Source: CAD feature listing. Evaluate the final solid. Frame: model axes, mm. Face numbers are marked on the shaded views. A direction names the side the tool comes from. Round coordinates to 2 decimals unless told otherwise and drop trailing zeros. Write each loop counter-clockwise with the first axis right and the second up, starting at its lowest first coordinate (ties: lowest second). Pieces come first, ordered by that corner, then holes. Notation, with made-up numbers: M 38.5,54 L 55.5,54 A19 cw 55.5,71 Z; hole C 2.5,13 d2. An arc over 180 degrees is marked long. Answer in a Markdown table with one row per item.
from build123d import *

# Parameters (mm, degrees)
SENSOR_BODY_BASE_DEPTH            = 9
CAMERA_HOLE_SKETCH_R              = 5.25
CAMERA_HOLE_DEPTH                 = 55.697637212
COVER_PLATE_CUTOUT_DEPTH          = 2
LED_DRIVER_CUTOUT_DEPTH           = 55.40433362
LED_DRIVER_CUTOUT_DEPTH_BACK      = 4
LEAD_START                        = 55.40433362
LEAD_CUTOUT_DEPTH                 = 62.40433362
FOLDED_LEAD_CUTOUT_DEPTH          = 4
GREEN_LEAD_CUTOUT_SKETCH_W        = 4
GREEN_LEAD_CUTOUT_SKETCH_H        = 6
GREEN_LEAD_CUTOUT_DEPTH           = 55.40433362
FOLDED_GREEN_LEAD_CUTOUT_SKETCH_W = 4.025
FOLDED_GREEN_LEAD_CUTOUT_SKETCH_H = 6
FOLDED_GREEN_LEAD_CUTOUT_DEPTH    = 4
CAMERA_PCB_CUTOUT_DEPTH           = 1.69
COVER_START                       = 1.69
COVER_PLATE_SUPPORT_DEPTH         = 1.69


with BuildPart() as part:
    # Sensor Body Base Sketch → Sensor Body Base (new body)
    with BuildSketch(Plane(origin=(0, 0, 0), x_dir=(1, 0, 0), z_dir=(0, 1, 0))):
        with BuildLine():
            Line((0, 17.5294293), (51.025, 17.5294293))
            Line((51.025, 17.5294293), (51.025, -17.5294293))
            Line((51.025, -17.5294293), (0, -17.5294293))
            ThreePointArc((0, -17.5294293), (-17.5294293, 0), (0, 17.5294293))
        make_face()
    extrude(amount=SENSOR_BODY_BASE_DEPTH)

    # Camera Hole Sketch → Camera Hole (cut, through all)
    with BuildSketch(Plane(origin=(0, 9, 0), x_dir=(1, 0, 0), z_dir=(0, 1, 0))):
        with Locations(Location((0, 0, 0), (0, 0, 270))):
            Circle(CAMERA_HOLE_SKETCH_R)
    extrude(amount=-CAMERA_HOLE_DEPTH, mode=Mode.SUBTRACT)

    # Cover Plate Cutout Sketch → Cover Plate Cutout (cut)
    # profile 1 of 2: a face of its own
    with BuildSketch(Plane(origin=(0, 9, 0), x_dir=(1, 0, 0), z_dir=(0, 1, 0))):
        with BuildLine():
            Line((47.325, 15.29), (0, 15.29))
            ThreePointArc((0, 15.29), (-15.29, 0), (0, -15.29))
            Line((0, -15.29), (47.325, -15.29))
            Line((47.325, -15.29), (47.325, -5.29))
            Line((47.325, -5.29), (47.325, 5.29))
            Line((47.325, 5.29), (47.325, 15.29))
        make_face()
        with BuildLine():
            ThreePointArc((4.308421985, -3), (-5.25, 0), (4.308421985, 3))
            Line((4.308421985, 3), (10.72655949, 3))
            Line((10.72655949, 3), (10.72655949, -3))
            Line((10.72655949, -3), (4.308421985, -3))
        make_face(mode=Mode.SUBTRACT)
    # profile 2 of 2: a face of its own
    with BuildSketch(Plane(origin=(0, 9, 0), x_dir=(1, 0, 0), z_dir=(0, 1, 0))):
        with BuildLine():
            Line((10.72655949, 3), (4.308421985, 3))
            ThreePointArc((4.308421985, 3), (5.009077531, 1.57214576), (5.25, 0))
            ThreePointArc((5.25, 0), (5.009077531, -1.57214576), (4.308421985, -3))
            Line((4.308421985, -3), (10.72655949, -3))
            Line((10.72655949, -3), (10.72655949, 3))
        make_face()
    extrude(amount=-COVER_PLATE_CUTOUT_DEPTH, mode=Mode.SUBTRACT)

    # LED Driver Cutout Sketch → LED Driver Cutout (cut, two sides: drawn at the far end of the back side and taken through both)
    with BuildSketch(Plane(origin=(0, 7, 0), x_dir=(1, 0, 0), z_dir=(0, 1, 0)).offset(-LED_DRIVER_CUTOUT_DEPTH_BACK)):
        Polygon((36.725, -17.5294293), (47.325, -17.5294293), (47.325, 17.5294293), (38.225, 17.5294293), (38.225, 15.29), (20.025, 15.29), (20.025, -15.29), (36.725, -15.29), align=None)
    extrude(amount=LED_DRIVER_CUTOUT_DEPTH + LED_DRIVER_CUTOUT_DEPTH_BACK, mode=Mode.SUBTRACT)

    # Cover Plate Fastener Sketch → Cover Plate Fastener (revolve, cut)
    with BuildSketch(Plane.XY, mode=Mode.PRIVATE) as cover_plate_fastener_sk:
        Polygon((8.5, 7), (8.5, 3.213974596), (10, 4.08), (10, 7), align=None)
    revolve(cover_plate_fastener_sk.sketch.rotate(Axis((8.5, 7, 0), (0, -1, 0)), 90), axis=Axis((8.5, 7, 0), (0, -1, 0)), mode=Mode.SUBTRACT)

    # Lead Cutout Shared Sketch → Lead Cutout (cut)
    with BuildSketch(Plane(origin=(0, 7, 0), x_dir=(1, 0, 0), z_dir=(0, 1, 0)).offset(LEAD_START)):
        with BuildLine():
            ThreePointArc((0, -13.5294293), (-6.76471465, -11.716829473), (-11.716829473, -6.76471465))
            Line((-11.716829473, -6.76471465), (-13.241528424, -7.645))
            ThreePointArc((-13.241528424, -7.645), (-7.645, -13.241528424), (0, -15.29))
            Line((0, -15.29), (11.279002615, -15.29))
            ThreePointArc((11.279002615, -15.29), (12.340917186, -14.446513871), (13.339960375, -13.5294293))
            Line((13.339960375, -13.5294293), (10.025, -13.5294293))
            Line((10.025, -13.5294293), (0, -13.5294293))
        make_face()
    lead_cutout = extrude(amount=-LEAD_CUTOUT_DEPTH, mode=Mode.SUBTRACT)

    # Sketch11<5> → Folded Lead Cutout (cut)
    with BuildSketch(Plane(origin=(0, 7, 0), x_dir=(1, 0, 0), z_dir=(0, 1, 0))):
        with BuildLine():
            Line((10.025, -4), (10.025, -13.5294293))
            Line((10.025, -13.5294293), (13.339960375, -13.5294293))
            ThreePointArc((13.339960375, -13.5294293), (13.687104196, -13.178132597), (14.025, -12.817931775))
            Line((14.025, -12.817931775), (14.025, -8))
            Line((14.025, -8), (20.025, -8))
            Line((20.025, -8), (20.025, -4))
            Line((20.025, -4), (10.025, -4))
        make_face()
    folded_lead_cutout = extrude(amount=-FOLDED_LEAD_CUTOUT_DEPTH, mode=Mode.SUBTRACT)

    # Lead Cutout Mirror: Lead Cutout, Folded Lead Cutout across plane
    add(lead_cutout.mirror(Plane.XY), mode=Mode.SUBTRACT)
    add(folded_lead_cutout.mirror(Plane.XY), mode=Mode.SUBTRACT)

    # Green Lead Cutout Sketch → Green Lead Cutout (cut, through all)
    with BuildSketch(Plane(origin=(0, 7, 0), x_dir=(1, 0, 0), z_dir=(0, 1, 0))):
        with Locations((14, 0)):
            Rectangle(GREEN_LEAD_CUTOUT_SKETCH_W, GREEN_LEAD_CUTOUT_SKETCH_H)
    extrude(amount=-GREEN_LEAD_CUTOUT_DEPTH, mode=Mode.SUBTRACT)

    # Folded Green Lead Cutout Sketch → Folded Green Lead Cutout (cut)
    with BuildSketch(Plane(origin=(0, 7, 0), x_dir=(1, 0, 0), z_dir=(0, 1, 0))):
        with Locations((18.0125, 0)):
            Rectangle(FOLDED_GREEN_LEAD_CUTOUT_SKETCH_W, FOLDED_GREEN_LEAD_CUTOUT_SKETCH_H)
    extrude(amount=-FOLDED_GREEN_LEAD_CUTOUT_DEPTH, mode=Mode.SUBTRACT)

    # Camera PCB Cutout Sketch → Camera PCB Cutout (cut)
    with BuildSketch(Plane(origin=(0, 7, 0), x_dir=(1, 0, 0), z_dir=(0, 1, 0))):
        with BuildLine():
            Line((-11.716829473, 6.76471465), (-13.241528424, 7.645))
            ThreePointArc((-13.241528424, 7.645), (-15.29, 0), (-13.241528424, -7.645))
            Line((-13.241528424, -7.645), (-11.716829473, -6.76471465))
            ThreePointArc((-11.716829473, -6.76471465), (-6.76471465, -11.716829473), (0, -13.5294293))
            Line((0, -13.5294293), (10.025, -13.5294293))
            Line((10.025, -13.5294293), (10.025, -4.5))
            Line((10.025, -4.5), (4.5, -4.5))
            Line((4.5, -4.5), (2.704163457, -4.5))
            ThreePointArc((2.704163457, -4.5), (0, -5.25), (-2.704163457, -4.5))
            Line((-2.704163457, -4.5), (-4.5, -4.5))
            Line((-4.5, -4.5), (-4.5, -2.704163457))
            ThreePointArc((-4.5, -2.704163457), (-5.25, 0), (-4.5, 2.704163457))
            Line((-4.5, 2.704163457), (-4.5, 4.5))
            Line((-4.5, 4.5), (-2.704163457, 4.5))
            ThreePointArc((-2.704163457, 4.5), (0, 5.25), (2.704163457, 4.5))
            Line((2.704163457, 4.5), (4.5, 4.5))
            Line((4.5, 4.5), (10.025, 4.5))
            Line((10.025, 4.5), (10.025, 13.5294293))
            Line((10.025, 13.5294293), (0, 13.5294293))
            ThreePointArc((0, 13.5294293), (-6.76471465, 11.716829473), (-11.716829473, 6.76471465))
        make_face()
        with BuildLine():
            Line((4.5, -4.5), (4.5, -2.704163457))
            ThreePointArc((4.5, -2.704163457), (3.712310601, -3.712310601), (2.704163457, -4.5))
            Line((2.704163457, -4.5), (4.5, -4.5))
        make_face()
        with BuildLine():
            ThreePointArc((-2.704163457, -4.5), (-3.712310601, -3.712310601), (-4.5, -2.704163457))
            Line((-4.5, -2.704163457), (-4.5, -4.5))
            Line((-4.5, -4.5), (-2.704163457, -4.5))
        make_face()
        with BuildLine():
            ThreePointArc((-4.5, 2.704163457), (-3.712310601, 3.712310601), (-2.704163457, 4.5))
            Line((-2.704163457, 4.5), (-4.5, 4.5))
            Line((-4.5, 4.5), (-4.5, 2.704163457))
        make_face()
        with BuildLine():
            Line((4.5, 2.704163457), (4.5, 4.5))
            Line((4.5, 4.5), (2.704163457, 4.5))
            ThreePointArc((2.704163457, 4.5), (3.712310601, 3.712310601), (4.5, 2.704163457))
        make_face()
    extrude(amount=-CAMERA_PCB_CUTOUT_DEPTH, mode=Mode.SUBTRACT)

    # Cover Plate Support Sketch → Cover Plate Support (add)
    with BuildSketch(Plane(origin=(0, 5.31, 0), x_dir=(1, 0, 0), z_dir=(0, 1, 0)).offset(COVER_START)):
        with BuildLine():
            Line((-11.716829473, 6.76471465), (-13.241528424, 7.645))
            ThreePointArc((-13.241528424, 7.645), (-15.29, 0), (-13.241528424, -7.645))
            Line((-13.241528424, -7.645), (-11.716829473, -6.76471465))
            ThreePointArc((-11.716829473, -6.76471465), (-13.5294293, 0), (-11.716829473, 6.76471465))
        make_face()
    extrude(amount=-COVER_PLATE_SUPPORT_DEPTH)


solid = part.part
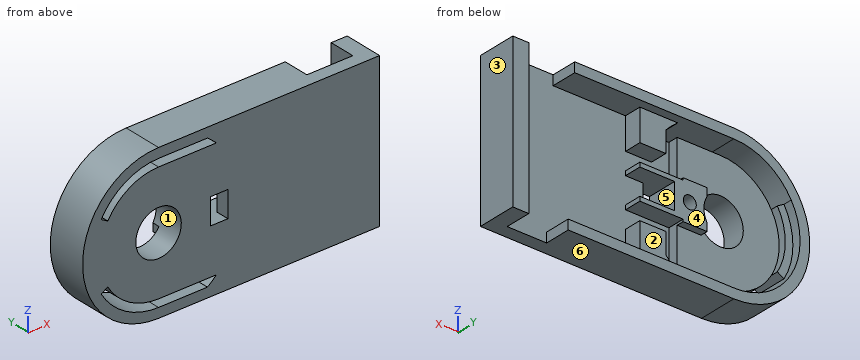
Q1. Access query for the marked faces 1 and 2. Directions: +Z, -Z, +X, -X, +Y, -Y. A direction counts if a zero-diameter tool reaches every point of the face in a straight line with its end or side. Return the directions, or none.
Solutions:
| item | result |
|---|---|
| face 1 | +Y, -Y |
| face 2 | +Y |
Q2. Material intervals for probe 1 along Z at (x, y) = (8.5, 6.2); probe 2 along Z at (x, y) = (8.5, 5.25); probe 3 along X at (y, z) = (5.5, 0) (3 decimals), sorted ascending.
Solutions:
| item | result |
|---|---|
| probe 1 | z = -17.53 to -15.29, -4.5 to -1.5, 1.5 to 4.5, 15.29 to 17.53 |
| probe 2 | z = -17.53 to -15.29, -13.53 to -1.5, 1.5 to 13.53, 15.29 to 17.53 |
| probe 3 | x = -17.529 to -13.529, 5.25 to 7, 10 to 12, 47.325 to 51.025 |
Q3. Section C-C (x = 31). Return loops of the section in (y, z), and give its area (3 significant figures).
Solutions:
| item | result |
|---|---|
| outline | M 0,-17.53 L 9,-17.53 L 9,-15.29 L 3,-15.29 L 3,15.29 L 9,15.29 L 9,17.53 L 0,17.53 Z |
| area | 132 mm2 |
Q4. Section B-B (z = 12). Return loops of the section in (x, y) (3 decimals), and give its area (3 significant figures).
Solutions:
| item | result |
|---|---|
| outline | M -12.778,0 L -9.475,0 L -9.475,9 L -12.778,9 Z; M -6.249,0 L 51.025,0 L 51.025,9 L 47.325,9 L 47.325,3 L 20.025,3 L 20.025,7 L 14.025,7 L 14.025,3 L 10.025,3 L 10.025,5.31 L -6.249,5.31 Z |
| area | 285 mm2 |
Q5. Pull-direction query (X, two-part tool) for the marked faces 3, 4, 5 and 6; classes: pulls with the +X half, pulls with the -X half, needs draft (parallel to the pull), parting line crosses it, or undercut.
Solutions:
| item | result |
|---|---|
| face 3 | pulls with the +X half |
| face 4 | undercut |
| face 5 | undercut |
| face 6 | needs draft |
Q6. Contact query for flat-ended pins moving along their axis: pin 1 Ø4.5 at (y, z) = (4.5, 11.5) entering from -X; pin 2 Ø8 at (x, z) = (41.5, -12) entering from +Y; pin 3 Ø3 at (y, z) = (4, -14) entering from -X. Output: stop coordinate, or through.
Solutions:
| item | result |
|---|---|
| pin 1 | stops at x = -14.89 |
| pin 2 | stops at y = 3 |
| pin 3 | stops at x = -12.29 |
Q7. Section A-A (y = 7.75). Return loops of the section in (x, z) (3 decimals), and give its area (3 significant figures).
Solutions:
| item | result |
|---|---|
| outline | M 0,-17.529 L 38.225,-17.529 L 38.225,-15.29 L 0,-15.29 A15.29 cw 0,15.29 L 36.725,15.29 L 36.725,17.529 L 0,17.529 A17.529 ccw Z; M 47.325,-17.529 L 51.025,-17.529 L 51.025,17.529 L 47.325,17.529 Z |
| area | 413 mm2 |
